Work out the finished part from the listing and answer in its coordinate system (mm). Round coordinates to 2 decimals unless told otherwise and drop trailing zeros. Write each loop counter-clockwise with the first axis right and the second up, starting at its lowest first coordinate (ties: lowest second). Pieces come first, ordered by that corner, then holes.
1. Find section A-A (x = -56.5). Write down the section's boundary in (y, z), and give its area (3 significant figures).
2. Find section B-B (y = 18). Write down the section's boundary in (x, z), and give its area (3 significant figures).
3. Find section C-C (z = 1.55). Write down the section's boundary in (x, y).
4. Flat-ended cylindrical pins translate along their axes: pin 1 Ø1.5 at (y, z) = (12.5, 2) entering from +X; pin 2 Ø1.5 at (y, z) = (13, 1.5) entering from -X. Find the tip coordinate at first contact, or state that the pin passes through.
5. Straight lines are drawn through the part: probe 1 along Y at (x, z) = (-58, 0.15); probe 2 along X at (y, z) = (5.5, 0.75); probe 3 along X at (y, z) = (6.5, 2.1). For each, find the intervals that lie inside material, in ascending order.
6. Find section D-D (y = 11). Write down the section's boundary in (x, z), and give its area (3 significant figures).
```python
from build123d import *

# Parameters (mm, degrees)
F1_DEPTH = 3
F3_DEPTH = 25
F4_ANGLE = 90
F5_ANGLE = -180


with BuildPart() as f1:
    # F0 (on Front) → F1 (new body)
    with BuildSketch(Plane.XZ):
        Polygon((66.5, 46), (46.5, 46), (30.8597909292, 30.5279652203), (32.9696138537, 28.395209438), (17.329404783, 12.9231746583), (15.2195818585, 15.0559304407), (0, 0), (113, 0), (97.7804181415, 15.0559304407), (95.670595217, 12.9231746583), (80.0303861463, 28.395209438), (82.1402090708, 30.5279652203), align=None)
    extrude(amount=F1_DEPTH)

    # F2 (on face) → F3 (cut)
    with BuildSketch(Plane.XZ.offset(3)):
        with BuildLine():
            Line((58.5, 10), (58.5, 19.6270607412))
            Line((58.5, 19.6270607412), (58.5, 20))
            ThreePointArc((58.5, 20), (56.5, 22), (54.5, 20))
            Line((54.5, 20), (54.5, 10))
            ThreePointArc((54.5, 10), (56.5, 8), (58.5, 10))
        make_face()
    extrude(amount=-F3_DEPTH, mode=Mode.SUBTRACT)


with BuildPart() as f1_1:
    # F4: moved
    add(f1.part.rotate(Axis((56.5, -3, 0), (1, 0, 0)), F4_ANGLE))


with BuildPart() as f1_2:
    # F5: moved
    add(f1_1.part.rotate(Axis((0, -3, 1.5), (0, 0, 1)), F5_ANGLE))


solid = f1_2.part
```
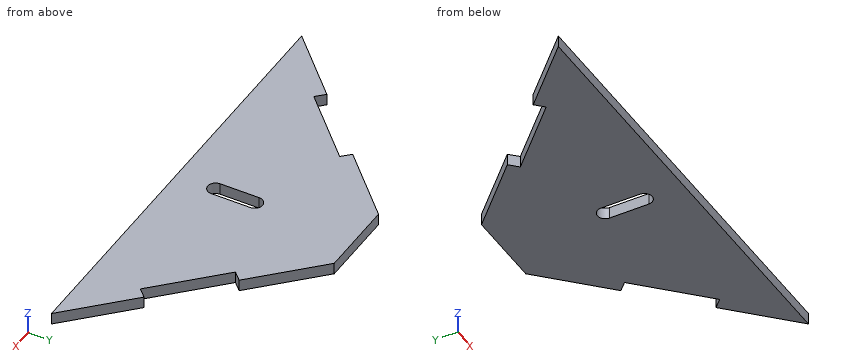
Worked answers:
1. outline: (-3, 0) - (5, 0) - (5, 3) - (-3, 3) - close; (19, 0) - (43, 0) - (43, 3) - (19, 3) - close
1. area: 96.0 mm2
2. outline: (-87.51, 0) - (-58.23, 0) - (-58.23, 3) - (-87.51, 3) - close; (-54.77, 0) - (-25.49, 0) - (-25.49, 3) - (-54.77, 3) - close
2. area: 176 mm2
3. outline: (-113, -3) - (0, -3) - (-15.22, 12.06) - (-17.33, 9.92) - (-32.97, 25.4) - (-30.86, 27.53) - (-46.5, 43) - (-66.5, 43) - (-82.14, 27.53) - (-80.03, 25.4) - (-95.67, 9.92) - (-97.78, 12.06) - close; hole (-58.5, 7) arc R2 ccw to (-54.5, 7) - (-54.5, 17) arc R2 ccw to (-58.5, 17) - close
4. pin 1: stops at x = -14.91
4. pin 2: stops at x = -93.32
5. probe 1: y = -3 to 5.68, 18.32 to 43
5. probe 2: x = -104.41 to -57.82, -55.18 to -8.59
5. probe 3: x = -103.4 to -58.44, -54.56 to -9.6
6. outline: (-98.85, 0) - (-96.74, 0) - (-96.74, 3) - (-98.85, 3) - close; (-94.58, 0) - (-58.5, 0) - (-58.5, 3) - (-94.58, 3) - close; (-54.5, 0) - (-18.42, 0) - (-18.42, 3) - (-54.5, 3) - close; (-16.26, 0) - (-14.15, 0) - (-14.15, 3) - (-16.26, 3) - close
6. area: 229 mm2
